from build123d import *

# Parameters (mm, degrees)
F1_DEPTH = 3


with BuildPart() as f1:
    # F0 (on Right) → F1 (new body)
    with BuildSketch(Plane.YZ):
        Polygon((-28.672605, -45.453316), (-28.672605, -48.453316), (-19.672605, -48.453316), (-27.672605, -39.453316), (-10.672605, 18.546684), (46.496383, 28.243702), (45.994689, 31.201455), (57.8257, 33.208234), (58.327395, 30.250482), (68.327395, 31.946684), (68.327395, 34.946684), (65.327395, 34.946684), (65.327395, 42.946684), (68.327395, 42.946684), (68.327395, 46.946684), (61.981544, 48.929763), (61.086719, 46.066323), (53.450879, 48.452523), (54.345704, 51.315963), (46.709864, 53.702163), (45.815039, 50.838723), (38.179199, 53.224923), (39.074024, 56.088362), (31.438184, 58.474562), (30.543359, 55.611122), (22.907519, 57.997322), (23.802344, 60.860762), (16.166505, 63.246962), (15.27168, 60.383522), (7.63584, 62.769722), (8.530665, 65.633162), (0.894825, 68.019362), (0, 65.155922), (-7.63584, 67.542122), (-6.741015, 70.405562), (-11.672605, 71.946684), (-21.672605, 71.946684), (-21.672605, 68.946684), (-37.672605, 68.946684), (-37.672605, 52.946684), (-34.672605, 52.946684), (-34.672605, 36.946684), (-37.672605, 36.946684), (-37.672605, 20.946684), (-34.672605, 20.946684), (-34.672605, 4.946684), (-37.672605, 4.946684), (-37.672605, -11.053316), (-34.672605, -11.053316), (-34.672605, -27.053316), (-37.672605, -27.053316), (-37.672605, -42.453316), (-34.672605, -42.453316), (-34.672605, -45.453316), align=None)
    extrude(amount=F1_DEPTH)


solid = f1.part
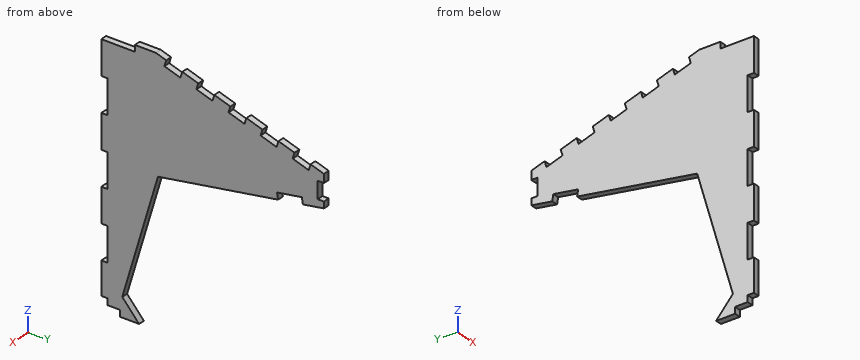
Check sheet for the modelled part. Datum: model origin and axes. Units: mm. Round coordinates to 2 decimals unless told otherwise and drop trailing zeros. Loops run counter-clockwise (first coordinate to the right, second up) from the corner with the lowest first, then second, coordinate; pieces in that order, holes last.
1. Sectioned sample at A-A on y = 51. Record the boundary of the cut face in (x, z).
2. Gauge pin test, flat ends, axial feed: pin 1 Ø1.5 at (x, y) = (1, -27) entering from +Z; pin 2 Ø1.5 at (x, y) = (2, 49) entering from +Z; pin 3 Ø0.9 at (x, y) = (2, 66.5) entering from +Z; pin 4 Ø3 at (y, z) = (-26.5, -17.5) entering from -X. Record the tip position at first contact, or that the pin passes through.
3. Scan lines: probe 1 along Y at (x, z) = (2.8, 41.5); probe 2 along Y at (x, z) = (2.15, 44); probe 3 along Z at (x, y) = (2.6, 10.5). Record each from-to range of solid material in increasing order.
4. Sectioned sample at B-B on z = 39. Record the boundary of the cut face in (x, y).
Recorded:
1. outline: (0, 32.05) - (3, 32.05) - (3, 52.36) - (0, 52.36) - close
2. pin 1: stops at z = 68.95
2. pin 2: stops at z = 53.22
2. pin 3: stops at z = 47.66
2. pin 4: stops at x = 0
3. probe 1: y = -34.67 to 65.33
3. probe 2: y = -34.67 to 68.33
3. probe 3: z = 22.14 to 61.87
4. outline: (0, -34.67) - (3, -34.67) - (3, 65.33) - (0, 65.33) - close
